Geometry: final body of the model. Coordinates: model frame, mm. Coordinates: 2 decimals unless noted, no trailing zeros. Loops run counter-clockwise (first coordinate to the right, second up) from the corner with the lowest first, then second, coordinate; pieces in that order, holes last. Notation, with made-up numbers: (46, 7.5) - (75, 7.5) arc R32 ccw to (75, 41.5) - close; hole circle Ø11 at (-36.75, 83.5). An arc over 180 degrees is marked (long way). Put each result on its own line as item: value. Start each with the question number.
1) Material intervals for line 1 along X through (y, z) = (12, 3.4) (3 decimals); line 2 along X through (y, z) = (16.5, 4.7) (3 decimals); line 3 along Y through (x, z) = (22.5, 2.65), sorted ascending. Write a range as from..to.
2) Contact query for flat-ended pins moving along their axis: pin 1 Ø1.5 at (y, z) = (15, 2.5) entering from +X; pin 2 Ø1.5 at (y, z) = (12.5, 2) entering from -X; pin 3 Ø1.5 at (y, z) = (18, 2.5) entering from -X; pin 4 Ø3 at (x, y) = (22.5, -2.5) entering from -Z. Output: stop coordinate, or through.
3) Section D-D on x = 22.5. Output: boundary loops of the cut face in (y, z).
4) Section C-C on x = -8.5. Output: boundary loops of the cut face in (y, z).
5) Section B-B on y = -2.5. Output: boundary loops of the cut face in (x, z).
6) Section A-A on z = 0.95. Output: boundary loops of the cut face in (x, y) (1 decimal).
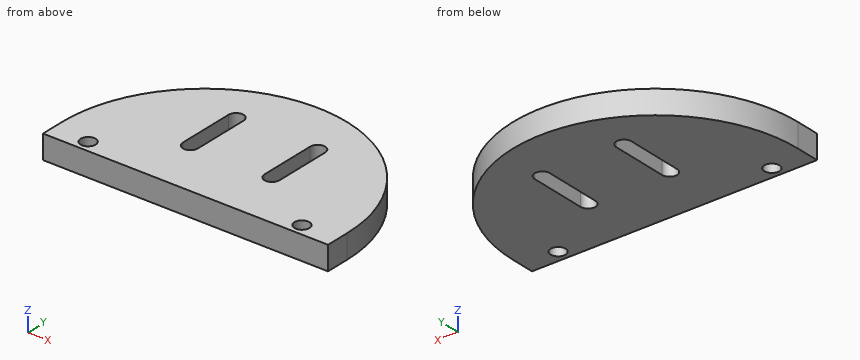
```python
from build123d import *

# Parameters (mm, degrees)
CROQUIS1_R              = 1.5875
SALIENTE_EXTRUIR1_DEPTH = 5


with BuildPart() as part:
    # Croquis1 → Saliente-Extruir1 (new body)
    with BuildSketch(Plane.XY):
        with BuildLine():
            Line((-30, 0), (-30, -5))
            Line((-30, -5), (30, -5))
            Line((30, -5), (30, 0))
            ThreePointArc((30, 0), (0, 30), (-30, 0))
        make_face()
        with Locations((-22.5, -2.5)):
            Circle(CROQUIS1_R, mode=Mode.SUBTRACT)
        with Locations((22.5, -2.5)):
            Circle(CROQUIS1_R, mode=Mode.SUBTRACT)
        with BuildLine():
            Line((-10.175, 7), (-10.175, 19))
            ThreePointArc((-10.175, 19), (-8.5875, 20.5875), (-7, 19))
            Line((-7, 19), (-7, 7))
            ThreePointArc((-7, 7), (-8.5875, 5.4125), (-10.175, 7))
        make_face(mode=Mode.SUBTRACT)
        with BuildLine():
            Line((7, 7), (7, 19))
            ThreePointArc((7, 19), (8.5875, 20.5875), (10.175, 19))
            Line((10.175, 19), (10.175, 7))
            ThreePointArc((10.175, 7), (8.5875, 5.4125), (7, 7))
        make_face(mode=Mode.SUBTRACT)
    extrude(amount=SALIENTE_EXTRUIR1_DEPTH)


solid = part.part
```
Answer block:
1. line 1: x = -27.495..-10.175, -7..7, 10.175..27.495
1. line 2: x = -25.055..-10.175, -7..7, 10.175..25.055
1. line 3: y = -5..-4.09, -0.91..19.84
2. pin 1: stops at x = 26.4
2. pin 2: stops at x = -27.6
2. pin 3: stops at x = -24.54
2. pin 4: passes through
3. outline: (-5, 0) - (-4.09, 0) - (-4.09, 5) - (-5, 5) - close; (-0.91, 0) - (19.84, 0) - (19.84, 5) - (-0.91, 5) - close
4. outline: (-5, 0) - (5.41, 0) - (5.41, 5) - (-5, 5) - close; (20.59, 0) - (28.77, 0) - (28.77, 5) - (20.59, 5) - close
5. outline: (-30, 0) - (-24.09, 0) - (-24.09, 5) - (-30, 5) - close; (-20.91, 0) - (20.91, 0) - (20.91, 5) - (-20.91, 5) - close; (24.09, 0) - (30, 0) - (30, 5) - (24.09, 5) - close
6. outline: (-30, -5) - (30, -5) - (30, 0) arc R30 ccw to (-30, 0) - close; hole circle Ø3.2 at (-22.5, -2.5); hole (-10.2, 7) arc R1.6 ccw to (-7, 7) - (-7, 19) arc R1.6 ccw to (-10.2, 19) - close; hole (7, 7) arc R1.6 ccw to (10.2, 7) - (10.2, 19) arc R1.6 ccw to (7, 19) - close; hole circle Ø3.2 at (22.5, -2.5)
